Geometry: final body of the model. Coordinates: model frame, mm. Give positions to 0.01 mm unless a question says otherwise; leave off trailing zeros. Order: outer loops, then holes, each group sorted by start corner. A loop starts at its lowest first (then second) coordinate and runs counter-clockwise, first axis right, second up. Notation, with made-up numbers: (47.5, 4) -> (87.5, 4) arc R13 cw to (87.5, 15) -> close; hole circle Ø1 at (55.5, 51). An arc over 180 degrees is marked (long way). Answer in a Markdown table with one row per item. Add a question column.
Q1. Cut plane D-D on z = -14.5. Return the cut outline in (x, y).
Q2. Cut plane B-B on x = 2.35. Return the cut outline in (y, z).
Q3. Cut plane C-C on z = 2.54. Return the cut outline in (x, y), and give its area (3 significant figures).
Q4. Line query: line 1 along Z through (x, y) = (1.8, 6.25); line 2 along Y through (x, z) = (1.05, -10.16); line 3 along Z through (x, y) = (1.05, 5.5). Output: solid intervals per line, ascending. Write a range as from..to.
Q5. Cut plane A-A on y = 6.35. Return the cut outline in (x, z), and give its area (3 significant figures).
from build123d import *

# Parameters (mm, degrees)
BOSS_EXTRUDE1_DEPTH   = 3.81
F_6_32_TAPPED_HOLE1_D = 2.7051
F_3_0MM_DOWEL_HOLE1_D = 3


with BuildPart() as part:
    # Sketch1 → Boss-Extrude1 (new body)
    with BuildSketch(Plane(origin=(0, 0, 0), x_dir=(0, 0, -1), z_dir=(1, 0, 0))):
        with BuildLine():
            Line((0, 0), (10.16, 0))
            ThreePointArc((10.16, 0), (16.51, 6.35), (10.16, 12.7))
            Line((10.16, 12.7), (0, 12.7))
            ThreePointArc((0, 12.7), (-6.35, 6.35), (0, 0))
        make_face()
    extrude(amount=BOSS_EXTRUDE1_DEPTH)

    # #6-32 Tapped Hole1 (through all)
    with Locations(Plane(origin=(3.81, 0, 0), x_dir=(0, 0, -1), z_dir=(1, 0, 0))):
        with Locations((-2.54, 6.35)):
            Hole(F_6_32_TAPPED_HOLE1_D / 2)

    # Ø3.0mm Dowel Hole1 (through all)
    with Locations(Plane(origin=(3.81, 0, 0), x_dir=(0, 0, -1), z_dir=(1, 0, 0))):
        with Locations((10.16, 6.35)):
            Hole(F_3_0MM_DOWEL_HOLE1_D / 2)


solid = part.part
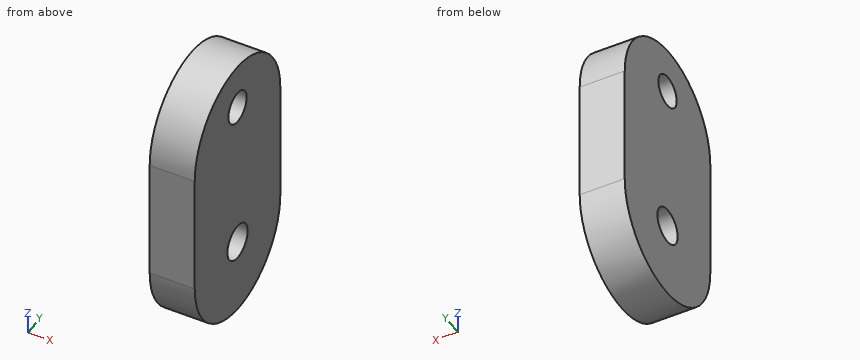
Completed:
| question | item | result |
|---|---|---|
| 1 | outline | (0, 1.71) -> (3.81, 1.71) -> (3.81, 10.99) -> (0, 10.99) -> close |
| 2 | outline | (0, -10.16) arc R6.35 ccw to (12.7, -10.16) -> (12.7, 0) arc R6.35 ccw to (0, 0) -> close; hole circle Ø3 at (6.35, -10.16); hole circle Ø2.71 at (6.35, 2.54) |
| 3 | outline | (0, 0.53) -> (3.81, 0.53) -> (3.81, 5) -> (0, 5) -> close; (0, 7.7) -> (3.81, 7.7) -> (3.81, 12.17) -> (0, 12.17) -> close |
| 3 | area | 34.0 mm² |
| 4 | line 1 | z = -16.51..-11.66, -8.66..1.19, 3.89..6.35 |
| 4 | line 2 | y = 0..4.85, 7.85..12.7 |
| 4 | line 3 | z = -16.45..-11.4, -8.92..1.49, 3.59..6.29 |
| 5 | outline | (0, -16.51) -> (3.81, -16.51) -> (3.81, -11.66) -> (0, -11.66) -> close; (0, -8.66) -> (3.81, -8.66) -> (3.81, 1.19) -> (0, 1.19) -> close; (0, 3.89) -> (3.81, 3.89) -> (3.81, 6.35) -> (0, 6.35) -> close |
| 5 | area | 65.4 mm² |
